from build123d import *

# Parameters (mm, degrees)
SKETCH1_W           = 5
SKETCH1_H           = 10.590486739
BOSS_EXTRUDE1_DEPTH = 15
SKETCH2_R           = 2.65
CUT_EXTRUDE1_DEPTH  = 23.048277791
SKETCH3_R           = 4.5
CUT_EXTRUDE2_DEPTH  = 5


with BuildPart() as part:
    # Sketch1 → Boss-Extrude1 (new body)
    with BuildSketch(Plane.XY):
        Polygon((20.353041123, 8.769305032), (10.103041123, 8.769305032), (0.103041123, -1.230694968), (0.103041123, -13.278972759), (10.103041123, -13.278972759), (16.560832175, -6.821181707), (18.353041123, -6.821181707), (18.353041123, -1.821181707), (20.353041123, -1.821181707), align=None)
        Polygon((25.353041123, -1.821181707), (20.353041123, -1.821181707), (18.353041123, -1.821181707), (18.353041123, -6.821181707), (27.353041123, -6.821181707), (27.353041123, -1.821181707), align=None)
        with Locations((22.853041123, 3.474061663)):
            Rectangle(SKETCH1_W, SKETCH1_H)
        Polygon((52.353041123, 8.769305032), (25.353041123, 8.769305032), (25.353041123, -1.821181707), (27.353041123, -1.821181707), (27.353041123, -6.821181707), (50.353041123, -6.821181707), (50.353041123, -1.821181707), (52.353041123, -1.821181707), align=None)
        Polygon((57.353041123, -1.821181707), (52.353041123, -1.821181707), (50.353041123, -1.821181707), (50.353041123, -6.821181707), (59.353041123, -6.821181707), (59.353041123, -1.821181707), align=None)
        with Locations((54.853041123, 3.474061663)):
            Rectangle(SKETCH1_W, SKETCH1_H)
        Polygon((67.603041123, 8.769305032), (57.353041123, 8.769305032), (57.353041123, -1.821181707), (59.353041123, -1.821181707), (59.353041123, -6.821181707), (61.145250072, -6.821181707), (67.603041123, -13.278972759), (77.603041123, -13.278972759), (77.603041123, -1.230694968), align=None)
    extrude(amount=BOSS_EXTRUDE1_DEPTH)

    # Sketch2 → Cut-Extrude1 (cut, through all)
    with BuildSketch(Plane(origin=(0, 8.769305032, 0), x_dir=(1, 0, 0), z_dir=(0, 1, 0))):
        with Locations((22.853041123, -7.5)):
            Circle(SKETCH2_R)
        with Locations((54.853041123, -7.5)):
            Circle(SKETCH2_R)
    extrude(amount=-CUT_EXTRUDE1_DEPTH, mode=Mode.SUBTRACT)

    # Sketch3 → Cut-Extrude2 (cut)
    with BuildSketch(Plane.XZ.offset(6.821181707)):
        with Locations((22.853041123, 7.5)):
            Circle(SKETCH3_R)
        with Locations((54.853041123, 7.5)):
            Circle(SKETCH3_R)
    extrude(amount=-CUT_EXTRUDE2_DEPTH, mode=Mode.SUBTRACT)


solid = part.part
Could you check a few things on this model? Use its own coordinates, in mm. A direction names the side the tool comes from. Round coordinates to 2 decimals unless told otherwise and drop trailing zeros. Write each loop counter-clockwise with the first axis right and the second up, starting at its lowest first coordinate (ties: lowest second). Pieces come first, ordered by that corner, then holes. Notation, with made-up numbers: (39, 66.25) - (65, 66.25) arc R18 ccw to (65, 86.25) - close; hole circle Ø10 at (53, 45.5). An arc over 180 degrees is marked (long way). Put each result on its own line as item: value. Start each with the question number.
(1) Thinking about a two-plate mould opening in X: for faces 1 (the flat face through (72.67, 3.7, 7.4)), 2 (the flat face through (54.8, -1.821, 4.6)), 3 (the flat face through (73, -13.279, 7)), 4 (the flat face through (5.173, 3.839, 7.395)), which applies, released by +X, released by -X, zero draft, split by the parting line, or undercut?
(2) For faces 5 (the flat face through (38, 0, 0)), 6 (the flat face through (64.329, -10.005, 7.395)), 7 (the flat face through (26, -1.821, 8)), which set-ups out of +Z, -Z, +X, -X, +Y, -Y let a thin tool reach every point of the face, with its end or its side?
(3) Will these pins go through, and if not, where does the flat tip stop? pin 1 (5 mm diameter, centred on x = 30.5, z = 8, fed in from -Y); pin 2 (3 mm diameter, centred on x = 54.85, z = 7.5, fed in from -Y); pin 3 (4.5 mm diameter, centred on x = 55, z = 6, fed in from -Y).
(4) I want a section at C-C, the plane y = -4. Please give me the cut outline in (x, z).
(5) I want a section at B-B, the plane x = 22.5. Please give me the cut outline in (y, z).
(6) I want a section at A-A, the plane z = 7.5. Please give me the cut outline in (x, y).
(7) I want a section at D-D, the plane y = -7.5. Please give me the cut outline in (x, z), plus the area to 3 significant figures.
(8) I need wall thicknesses on probe 1 along X at (y, z) = (-3.25, 8.5); probe 2 along X at (y, z) = (0.75, 9); probe 3 along Y at (x, z) = (31, 4.75). Which ranges of each line are inside material? Lowest first, please.
Here are the results:
1. face 1: released by +X
1. face 2: undercut
1. face 3: zero draft
1. face 4: released by -X
2. face 5: -Z, +X, -X, +Y, -Y
2. face 6: +Z, -Z, -Y
2. face 7: -Y
3. pin 1: stops at y = -6.82
3. pin 2: passes through
3. pin 3: stops at y = -1.82
4. outline: (0.1, 0) - (77.6, 0) - (77.6, 15) - (0.1, 15) - close; hole circle Ø9 at (22.85, 7.5); hole circle Ø9 at (54.85, 7.5)
5. outline: (-6.82, 0) - (8.77, 0) - (8.77, 4.87) - (-1.82, 4.87) - (-1.82, 3.01) - (-6.82, 3.01) - close; (-6.82, 11.99) - (-1.82, 11.99) - (-1.82, 10.13) - (8.77, 10.13) - (8.77, 15) - (-6.82, 15) - close
6. outline: (0.1, -13.28) - (10.1, -13.28) - (16.56, -6.82) - (18.35, -6.82) - (18.35, -1.82) - (20.2, -1.82) - (20.2, 8.77) - (10.1, 8.77) - (0.1, -1.23) - close; (25.5, -1.82) - (27.35, -1.82) - (27.35, -6.82) - (50.35, -6.82) - (50.35, -1.82) - (52.2, -1.82) - (52.2, 8.77) - (25.5, 8.77) - close; (57.5, -1.82) - (59.35, -1.82) - (59.35, -6.82) - (61.15, -6.82) - (67.6, -13.28) - (77.6, -13.28) - (77.6, -1.23) - (67.6, 8.77) - (57.5, 8.77) - close
7. outline: (0.1, 0) - (15.88, 0) - (15.88, 15) - (0.1, 15) - close; (61.82, 0) - (77.6, 0) - (77.6, 15) - (61.82, 15) - close
7. area: 473 mm^2
8. probe 1: x = 0.1 to 18.47, 27.24 to 50.47, 59.24 to 77.6
8. probe 2: x = 2.08 to 20.67, 25.04 to 52.67, 57.04 to 75.62
8. probe 3: y = -6.82 to 8.77
